Geometry check sheet. Reference: the model listing, model coordinates, mm. Face numbers are marked on the shaded views. A direction names the side the tool comes from. Coordinates: 2 decimals unless noted, no trailing zeros. Loops run counter-clockwise (first coordinate to the right, second up) from the corner with the lowest first, then second, coordinate; pieces in that order, holes last.
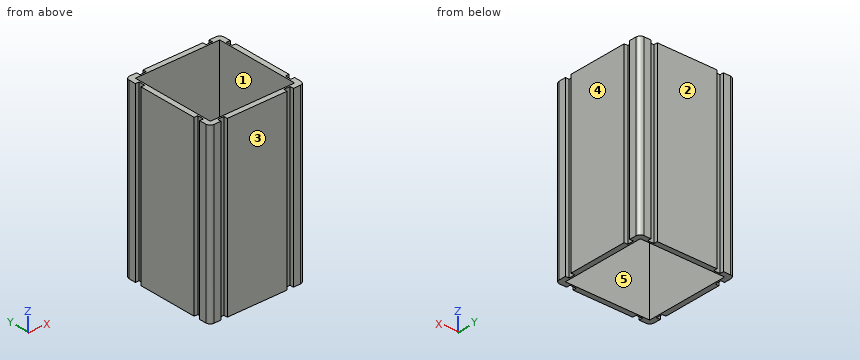
from build123d import *

# Parameters (mm, degrees)
F0_W            = 40
F0_H            = 40
F1_DEPTH        = 82
F2_W            = 3
F2_H            = 1.75
F3_DEPTH        = 82
F3_COPIES_COUNT = 4


# Not quite as in the source:
# - a pattern or mirror of a feature is missing from the dataset's text; its kind, count and spacing are read off the source's solid


with BuildPart() as f1:
    # F0 (on Top) → F1 (new body)
    with BuildSketch(Plane.XY):
        with BuildLine():
            Line((-20.5, -22.5), (20.5, -22.5))
            ThreePointArc((20.5, -22.5), (21.9142135624, -21.9142135624), (22.5, -20.5))
            Line((22.5, -20.5), (22.5, 20.5))
            ThreePointArc((22.5, 20.5), (21.9142135624, 21.9142135624), (20.5, 22.5))
            Line((20.5, 22.5), (-20.5, 22.5))
            ThreePointArc((-20.5, 22.5), (-21.9142135624, 21.9142135624), (-22.5, 20.5))
            Line((-22.5, 20.5), (-22.5, -20.5))
            ThreePointArc((-22.5, -20.5), (-21.9142135624, -21.9142135624), (-20.5, -22.5))
        make_face()
        Rectangle(F0_W, F0_H, mode=Mode.SUBTRACT)
    extrude(amount=F1_DEPTH)

    # F2 (on face) → F3 (cut, through all)
    with BuildSketch(Plane.XY.offset(82)):
        with Locations((-15.68, 21.625)):
            Rectangle(F2_W, F2_H)
        with Locations((15.68, 21.625)):
            Rectangle(F2_W, F2_H)
    f3 = extrude(amount=-F3_DEPTH, mode=Mode.SUBTRACT)

    # F3_copies: F3 ×4 about axis
    f3_copies_axis = Axis((0, 0, 0), (0, 0, 1))
    for i in range(1, F3_COPIES_COUNT):
        add(f3.rotate(f3_copies_axis, i * 360 / F3_COPIES_COUNT), mode=Mode.SUBTRACT)


solid = f1.part
(1) Gauge pin test, flat ends, axial feed: pin 1 Ø0.9 at (x, z) = (21.5, 61.5) entering from -Y; pin 2 Ø0.5 at (x, z) = (21.5, 30.5) entering from +Y; pin 3 Ø0.5 at (y, z) = (-21.5, 32) entering from +X. Record the tip position at first contact, or that the pin passes through.
Findings:
pin 1: stops at y = -22.42
pin 2: stops at y = 22.35
pin 3: stops at x = 22.35
(2) Scan lines: L1, parallel to X at y = 9, z = 43.5; L2, parallel to X at y = -14.5, z = 19.5. Record each from-to range of solid material in increasing order.
Findings:
L1: x = -22.5 to -20, 20 to 22.5
L2: x = -20.75 to -20, 20 to 20.75
(3) Sectioned sample at A-A on x = -1. Record the cut outline in (y, z).
Findings:
outline: (-22.5, 0) - (-20, 0) - (-20, 82) - (-22.5, 82) - close; (20, 0) - (22.5, 0) - (22.5, 82) - (20, 82) - close
(4) Draft check along Y on the marked faces 3, 4 and 5. Enter one of: +Y half, -Y half, draft (parallel to the pull), parting line (faces both ways), or undercut.
Findings:
face 3: -Y half
face 4: draft
face 5: undercut
(5) Sectioned sample at B-B on y = -16. Record the cut outline in (x, z).
Findings:
outline: (-20.75, 0) - (-20, 0) - (-20, 82) - (-20.75, 82) - close; (20, 0) - (20.75, 0) - (20.75, 82) - (20, 82) - close
(6) Access from +Z, -Z, +X, -X, +Y, -Y to the whole of each face (thin tool, end or side, straight path). Record for the marked faces 1 and 2.
Findings:
face 1: +Z, -Z
face 2: +Z, -Z, +X, -X, +Y
